from build123d import *

# Parameters (mm, degrees)
SKETCH_1_W          = 8
SKETCH_1_H          = 35
EXTRUDE_1_DEPTH     = 60
CUT_EXTRUDE_1_DEPTH = 60
SKETCH_3_R          = 2.1
CUT_EXTRUDE_2_DEPTH = 10
SKETCH_4_R          = 4.05
CUT_EXTRUDE_3_DEPTH = 46
SKETCH_5_R          = 2.1
CUT_EXTRUDE_4_DEPTH = 10
SKETCH_7_R          = 4.05
EXTRUDE_2_DEPTH     = 2


with BuildPart() as part:
    # 草图1 → 凸台-拉伸1 (new body)
    with BuildSketch(Plane(origin=(0, 0, 0), x_dir=(1, 0, 0), z_dir=(0, 1, 0))):
        Rectangle(SKETCH_1_W, SKETCH_1_H)
    extrude(amount=EXTRUDE_1_DEPTH)

    # 草图2 → 切除-拉伸1 (cut)
    with BuildSketch(Plane(origin=(4, 0, 0), x_dir=(0, 0, -1), z_dir=(1, 0, 0))):
        with BuildLine():
            Line((-17.5, 15), (-9.450518874, 38.269203727))
            ThreePointArc((-9.450518874, 38.269203727), (-1.17e-07, 45), (9.450518798, 38.269203948))
            Line((9.450518798, 38.269203948), (17.5, 15))
            Line((17.5, 15), (17.5, 60))
            Line((17.5, 60), (-17.5, 60))
            Line((-17.5, 60), (-17.5, 15))
        make_face()
    extrude(amount=-CUT_EXTRUDE_1_DEPTH, mode=Mode.SUBTRACT)

    # 草图3 → 切除-拉伸2 (cut)
    with BuildSketch(Plane.XZ):
        with Locations(Location((0, -12.5, 0), (0, 0, 270))):
            Circle(SKETCH_3_R)
        with Locations(Location((0, 12.5, 0), (0, 0, 270))):
            Circle(SKETCH_3_R)
    extrude(amount=-CUT_EXTRUDE_2_DEPTH, mode=Mode.SUBTRACT)

    # 草图4 → 切除-拉伸3 (cut)
    with BuildSketch(Plane(origin=(4, 0, 0), x_dir=(0, 0, -1), z_dir=(1, 0, 0))):
        with Locations((0, 35)):
            Circle(SKETCH_4_R)
    extrude(amount=-CUT_EXTRUDE_3_DEPTH, mode=Mode.SUBTRACT)

    # 草图5 → 切除-拉伸4 (cut)
    with BuildSketch(Plane.ZY.offset(4)):
        with Locations((10, 20)):
            Circle(SKETCH_5_R)
        with Locations((-10, 20)):
            Circle(SKETCH_5_R)
        with Locations((5, 5)):
            Circle(SKETCH_5_R)
        with Locations((-5, 5)):
            Circle(SKETCH_5_R)
    extrude(amount=-CUT_EXTRUDE_4_DEPTH, mode=Mode.SUBTRACT)


with BuildPart() as body_2:
    # 草图7 → 凸台-拉伸2 (new body)
    with BuildSketch(Plane.ZY.offset(4)):
        with Locations(Location((0, 35, 0), (0, 0, 180))):
            Circle(SKETCH_7_R)
    extrude(amount=-EXTRUDE_2_DEPTH)

    # Combine 3: union part
    add(part.part)


solid = body_2.part
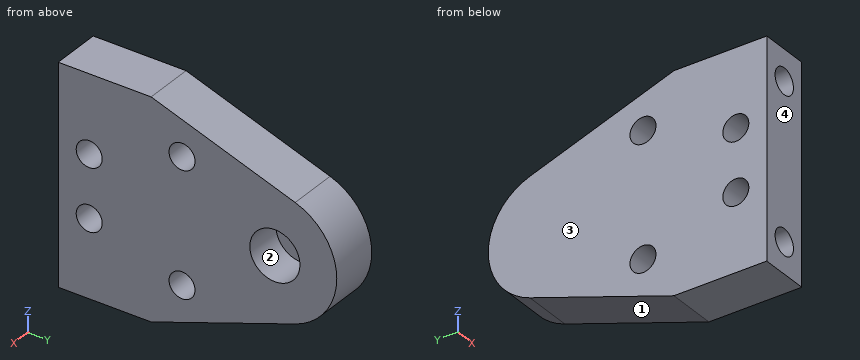
The listing builds one solid part. Answer for the finished solid, in the listing's coordinates (mm). Face numbers are marked on the shaded views. Give positions to 0.01 mm unless a question says otherwise; leave off trailing zeros. Write each loop counter-clockwise with the first axis right and the second up, starting at its lowest first coordinate (ties: lowest second). Pieces come first, ordered by that corner, then holes. Notation, with made-up numbers: (80.25, 15) -> (130.25, 15) arc R16 ccw to (130.25, 21) -> close; hole circle Ø1 at (40, 27). An arc over 180 degrees is marked (long way). Use a Markdown table: item, result.
(1) Section A-A, the plane x = 0 is taken. Determine the outline of the cut face in (y, z), then the cut area to 3 significant figures.
Return value:
| item | result |
|---|---|
| outline | (0, -17.5) -> (15, -17.5) -> (38.27, -9.45) arc R10 ccw to (38.27, 9.45) -> (15, 17.5) -> (0, 17.5) -> (0, 14.6) -> (10, 14.6) -> (10, 10.4) -> (0, 10.4) -> (0, -10.4) -> (10, -10.4) -> (10, -14.6) -> (0, -14.6) -> close; hole circle Ø4.2 at (5, -5); hole circle Ø4.2 at (5, 5); hole circle Ø4.2 at (20, -10); hole circle Ø4.2 at (20, 10); hole circle Ø8.1 at (35, 0) |
| area | 1,050 mm2 |
(2) Flat-ended cylindrical pins translate along their axes: P1, Ø7.5, axis at y = 35, z = 0, coming from the +X side; P2, Ø1.3, axis at x = 0.5, z = 11.5, coming from the -Y side. Find the tip coordinate at first contact, or state that the pin passes through.
Return value:
| item | result |
|---|---|
| P1 | x = -2 |
| P2 | y = 10 |
(3) Section D-D, the plane y = 6 is taken. Determine the outline of the cut face in (x, z), then the cut area to 3 significant figures.
Return value:
| item | result |
|---|---|
| outline | (-4, -17.5) -> (4, -17.5) -> (4, -6.85) -> (-4, -6.85) -> close; (-4, -3.15) -> (4, -3.15) -> (4, 3.15) -> (-4, 3.15) -> close; (-4, 6.85) -> (4, 6.85) -> (4, 17.5) -> (-4, 17.5) -> close; hole circle Ø4.2 at (0, -12.5); hole circle Ø4.2 at (0, 12.5) |
| area | 193 mm2 |
(4) Determine the mould class of the marked faces 1, 2, 3 and 4 for opening direction Y: released by +Y, released by -Y, zero draft, split by the parting line, or undercut.
Return value:
| item | result |
|---|---|
| face 1 | released by +Y |
| face 2 | undercut |
| face 3 | zero draft |
| face 4 | released by -Y |
(5) Section B-B, the plane x = -3.5 is taken. Determine the outline of the cut face in (y, z).
Return value:
| item | result |
|---|---|
| outline | (0, -17.5) -> (15, -17.5) -> (38.27, -9.45) arc R10 ccw to (38.27, 9.45) -> (15, 17.5) -> (0, 17.5) -> close; hole circle Ø4.2 at (5, -5); hole circle Ø4.2 at (5, 5); hole circle Ø4.2 at (20, -10); hole circle Ø4.2 at (20, 10) |
(6) Find the intervals of material crossed by probe 1 along X at (y, z) = (3.5, 12.5); probe 2 along Y at (x, z) = (2.25, -8.5); probe 3 along Y at (x, z) = (0, 0.5), in increasing order. Write a range as from..to.
Return value:
| item | result |
|---|---|
| probe 1 | -4..-2.1, 2.1..4 |
| probe 2 | 0..18.53, 21.47..40.27 |
| probe 3 | 0..30.98, 39.02..44.99 |
(7) Section C-C, the plane z = 11 is taken. Determine the outline of the cut face in (x, y), then the cut area to 3 significant figures.
Return value:
| item | result |
|---|---|
| outline | (-4, 0) -> (-1.47, 0) -> (-1.47, 10) -> (1.47, 10) -> (1.47, 0) -> (4, 0) -> (4, 18.15) -> (-4, 18.15) -> close; (-4, 21.85) -> (4, 21.85) -> (4, 33.79) -> (-4, 33.79) -> close |
| area | 211 mm2 |
